```python
from build123d import *

# Parameters (mm, degrees)
F0_W         = 25
F0_H         = 10
F1_DEPTH     = 8
F2_W         = 25
F2_H         = 10
F3_DEPTH     = 0.7
F4_R         = 1
F5_T1_DEPTH  = 10.2
F5_S5_W      = 1
F5_S5_H      = 1
F5_T6_DEPTH  = 1
F6_T1_DEPTH  = 10.2
F6_S5_W      = 1
F6_S5_H      = 1
F6_T6_DEPTH  = 1
F6_S11_W     = 1
F6_S11_H     = 1
F6_T12_DEPTH = 1
F6_S17_W     = 1
F6_S17_H     = 1
F6_T18_DEPTH = 1


# Not quite as in the source:
# - a fillet or chamfer that OpenCascade refuses, or shapes differently, is made with other operations: its cross-section is extruded or revolved along the edge and cut away or added


with BuildPart() as f1:
    # F0 (on Top) → F1 (new body)
    with BuildSketch(Plane.XY):
        Rectangle(F0_W, F0_H)
        Polygon((-10, 2.45), (10, 2.45), (10, -2.45), (10, -3.65), (6.8, -3.65), (6.8, -2.45), (-6.8, -2.45), (-6.8, -3.65), (-10, -3.65), (-10, -2.45), align=None, mode=Mode.SUBTRACT)
    extrude(amount=F1_DEPTH)

    # F2 (on face) → F3 (join)
    with BuildSketch(Plane.XY.offset(8)):
        Rectangle(F2_W, F2_H)
    extrude(amount=F3_DEPTH)

    # F4
    f4_edges = [f1.edges().sort_by_distance(p)[0] for p in [
        (0, 5, 8.7),
        (-12.5, 0, 8.7),
        (0, -5, 8.7),
        (12.5, 0, 8.7),
    ]]
    fillet(f4_edges, radius=F4_R)

    # F5: fillet of radius 1 on 1 edges, made by hand

    # F5_s2 → F5_t1 (cut)
    with BuildSketch(Plane.XY.offset(-2.5)):
        with BuildLine():
            ThreePointArc((12.5, 4), (12.2071067812, 4.7071067812), (11.5, 5))
            Line((11.5, 5), (12.5, 5))
            Line((12.5, 5), (12.5, 4))
        make_face()
    extrude(amount=F5_T1_DEPTH, mode=Mode.SUBTRACT)


with BuildPart() as f5_tool4:
    # F5_s5 → F5_t6 (new body)
    with BuildSketch(Plane.YZ.offset(11.5)):
        with Locations((4.5, 8.2)):
            Rectangle(F5_S5_W, F5_S5_H)
    extrude(amount=F5_T6_DEPTH)

    # F5_s7 → F5_t8 (revolve, cut)
    with BuildSketch(Plane(origin=(11.5, 4, 7.7), x_dir=(0, -0.7071067812, -0.7071067812), z_dir=(0, -0.7071067812, 0.7071067812))):
        with BuildLine():
            ThreePointArc((0, -1), (1, 0), (0, 1))
            Line((0, 1), (0, -1))
        make_face()
    revolve(axis=Axis((11.5, 4, 7.7), (1, 0, 0)), mode=Mode.SUBTRACT)


with BuildPart() as f1_1:
    add(f1.part)

    # F5_t3: cut F5_tool4
    add(f5_tool4.part, mode=Mode.SUBTRACT)

    # F6: fillet of radius 1 on 3 edges, made by hand

    # F6_s2 → F6_t1 (cut)
    with BuildSketch(Plane.XY.offset(-2.5)):
        with BuildLine():
            ThreePointArc((-12.5, 4), (-12.2071067812, 4.7071067812), (-11.5, 5))
            Line((-11.5, 5), (-12.5, 5))
            Line((-12.5, 5), (-12.5, 4))
        make_face()
        with BuildLine():
            ThreePointArc((11.5, -5), (12.2071067812, -4.7071067812), (12.5, -4))
            Line((12.5, -4), (12.5, -5))
            Line((12.5, -5), (11.5, -5))
        make_face()
        with BuildLine():
            ThreePointArc((-11.5, -5), (-12.2071067812, -4.7071067812), (-12.5, -4))
            Line((-12.5, -4), (-12.5, -5))
            Line((-12.5, -5), (-11.5, -5))
        make_face()
    extrude(amount=F6_T1_DEPTH, mode=Mode.SUBTRACT)


with BuildPart() as f6_tool4:
    # F6_s5 → F6_t6 (new body)
    with BuildSketch(Plane.XZ.offset(4)):
        with Locations((-12, 8.2)):
            Rectangle(F6_S5_W, F6_S5_H)
    extrude(amount=F6_T6_DEPTH)

    # F6_s7 → F6_t8 (revolve, cut)
    with BuildSketch(Plane(origin=(-11.5, -4, 7.7), x_dir=(0.7071067812, 0, -0.7071067812), z_dir=(-0.7071067812, 0, -0.7071067812))):
        with BuildLine():
            ThreePointArc((0, -1), (1, 0), (0, 1))
            Line((0, 1), (0, -1))
        make_face()
    revolve(axis=Axis((-11.5, -4, 7.7), (0, -1, 0)), mode=Mode.SUBTRACT)


with BuildPart() as f1_2:
    add(f1_1.part)

    # F6_t3: cut F6_tool4
    add(f6_tool4.part, mode=Mode.SUBTRACT)


with BuildPart() as f6_tool10:
    # F6_s11 → F6_t12 (new body)
    with BuildSketch(Plane.XZ.offset(4)):
        with Locations((12, 8.2)):
            Rectangle(F6_S11_W, F6_S11_H)
    extrude(amount=F6_T12_DEPTH)

    # F6_s13 → F6_t14 (revolve, cut)
    with BuildSketch(Plane(origin=(11.5, -4, 7.7), x_dir=(-0.7071067812, 0, -0.7071067812), z_dir=(-0.7071067812, 0, 0.7071067812))):
        with BuildLine():
            ThreePointArc((0, -1), (1, 0), (0, 1))
            Line((0, 1), (0, -1))
        make_face()
    revolve(axis=Axis((11.5, -4, 7.7), (0, -1, 0)), mode=Mode.SUBTRACT)


with BuildPart() as f1_3:
    add(f1_2.part)

    # F6_t9: cut F6_tool10
    add(f6_tool10.part, mode=Mode.SUBTRACT)


with BuildPart() as f6_tool16:
    # F6_s17 → F6_t18 (new body)
    with BuildSketch(Plane.YZ.offset(-11.5)):
        with Locations((4.5, 8.2)):
            Rectangle(F6_S17_W, F6_S17_H)
    extrude(amount=-F6_T18_DEPTH)

    # F6_s19 → F6_t20 (revolve, cut)
    with BuildSketch(Plane(origin=(-11.5, 4, 7.7), x_dir=(0, -0.7071067812, -0.7071067812), z_dir=(0, 0.7071067812, -0.7071067812))):
        with BuildLine():
            ThreePointArc((0, -1), (1, 0), (0, 1))
            Line((0, 1), (0, -1))
        make_face()
    revolve(axis=Axis((-11.5, 4, 7.7), (-1, 0, 0)), mode=Mode.SUBTRACT)


with BuildPart() as f1_4:
    add(f1_3.part)

    # F6_t15: cut F6_tool16
    add(f6_tool16.part, mode=Mode.SUBTRACT)


solid = f1_4.part
```
Model file for the job. Use its own axes, mm. A direction names the side the tool comes from. Round coordinates to 2 decimals unless told otherwise and drop trailing zeros. Write each loop counter-clockwise with the first axis right and the second up, starting at its lowest first coordinate (ties: lowest second). Pieces come first, ordered by that corner, then holes. Notation, with made-up numbers: (-16, 43) -> (38, 43) arc R20 ccw to (38, 63) -> close; hole circle Ø10 at (43, -1). An arc over 180 degrees is marked (long way). Answer as CSV lines item,"result".
1. Mould opens along Y. For faces 1 (the face through (-8, -3.65, 4)), 2 (the face through (-10, -1, 4)), 3 (the face through (0, 3, 0)), 4 (the face through (-12.215, 4.699, 3.796)) say: +Y half, -Y half, draft (parallel to the pull), parting line (faces both ways), or undercut.
Resolved:
face 1,"undercut"
face 2,"undercut"
face 3,"draft"
face 4,"+Y half"
2. Slice it at C-C, the plane x = 3.5. List the corners of the cut face in (y, z).
Resolved:
outline,"(-5, 0) -> (-2.45, 0) -> (-2.45, 8) -> (2.45, 8) -> (2.45, 0) -> (5, 0) -> (5, 7.7) arc R1 ccw to (4, 8.7) -> (-4, 8.7) arc R1 ccw to (-5, 7.7) -> close"
3. Tool access for faces 5 (the face through (12.5, 0, 4)), 6 (the face through (-6.8, -3, 4)): list every direction of +Z, -Z, +X, -X, +Y, -Y with a clear straight run to the whole face (end or side of a thin tool).
Resolved:
face 5,"+Z, -Z, +X, +Y, -Y"
face 6,"-Z"
4. Slice it at A-A, the plane z = 6. List the corners of the cut face in (x, y).
Resolved:
outline,"(-12.5, -4) arc R1 ccw to (-11.5, -5) -> (11.5, -5) arc R1 ccw to (12.5, -4) -> (12.5, 4) arc R1 ccw to (11.5, 5) -> (-11.5, 5) arc R1 ccw to (-12.5, 4) -> close; hole (-10, -3.65) -> (-6.8, -3.65) -> (-6.8, -2.45) -> (6.8, -2.45) -> (6.8, -3.65) -> (10, -3.65) -> (10, 2.45) -> (-10, 2.45) -> close"
5. Slice it at D-D, the plane y = 0.75. List the corners of the cut face in (x, z).
Resolved:
outline,"(-12.5, 0) -> (-10, 0) -> (-10, 8) -> (10, 8) -> (10, 0) -> (12.5, 0) -> (12.5, 7.7) arc R1 ccw to (11.5, 8.7) -> (-11.5, 8.7) arc R1 ccw to (-12.5, 7.7) -> close"
6. Pin check, flat tip, straight feed: pin 1 Ø1.5 at (x, y) = (4, -1.5) entering from -Z. Stop position of the tip, or through.
Resolved:
pin 1,"z = 8"
7. Slice it at B-B, the plane y = -3. List the corners of the cut face in (x, z), plus the area to 3 significant figures.
Resolved:
outline,"(-12.5, 0) -> (-10, 0) -> (-10, 8) -> (-6.8, 8) -> (-6.8, 0) -> (6.8, 0) -> (6.8, 8) -> (10, 8) -> (10, 0) -> (12.5, 0) -> (12.5, 7.7) arc R1 ccw to (11.5, 8.7) -> (-11.5, 8.7) arc R1 ccw to (-12.5, 7.7) -> close"
area,"166 mm²"
8. Drill centre lines: line 1 (X direction, y = -3.5, z = 3); line 2 (Y direction, x = -6, z = 7.25); line 3 (X direction, y = 1.25, z = 6). Where is each one in solid material? Low to high.
Resolved:
line 1,"-12.5 to -10, -6.8 to 6.8, 10 to 12.5"
line 2,"-5 to -2.45, 2.45 to 5"
line 3,"-12.5 to -10, 10 to 12.5"
